```python
from build123d import *

# Parameters (mm, degrees)
F0_R     = 25.4
F0_R_2   = 12.7
F1_DEPTH = 3.175
F2_R     = 12.7
F3_DEPTH = 12.7


with BuildPart() as f1:
    # F0 (on Front) → F1 (new body)
    with BuildSketch(Plane.XZ):
        with Locations((-49.276002, 2.029355)):
            Circle(F0_R)
        with Locations((-49.276002, 2.029355)):
            Circle(F0_R_2, mode=Mode.SUBTRACT)
    extrude(amount=F1_DEPTH)

    # F2 (on face) → F3 (join)
    with BuildSketch(Plane.XZ.offset(3.175)):
        Polygon((-39.038599, -21.216195), (-24.026064, -0.727569), (-34.263467, 22.517981), (-59.513405, 25.274904), (-74.52594, 4.786278), (-64.288537, -18.459271), align=None)
        with Locations((-49.276002, 2.029355)):
            Circle(F2_R, mode=Mode.SUBTRACT)
    extrude(amount=F3_DEPTH)


solid = f1.part
```
Source: CAD feature listing. Evaluate the final solid. Frame: model axes, mm. A direction names the side the tool comes from. Coordinates: 2 decimals unless noted, no trailing zeros. Order: outer loops, then holes, each group sorted by start corner. A loop starts at its lowest first (then second) coordinate and runs counter-clockwise, first axis right, second up. Notation, with made-up numbers: (10.25, 75.5) - (68.25, 75.5) arc R16 ccw to (68.25, 94.5) - close; hole circle Ø2 at (40.25, 60). An arc over 180 degrees is marked (long way). One line per item, written item: value.
1) Ray query, line 1 (X direction, y = -11.5, z = -6); line 2 (Z direction, x = -42, y = -2.5); line 3 (Y direction, x = -28, z = -8.5) (3 decimals). Return the intervals inside material, ascending. Write a range as [from, to].
Computed values:
line 1: x = [-69.78, -59.12], [-39.44, -27.89]
line 2: z = [-22.31, -8.38], [12.44, 26.36]
line 3: y = [-3.175, 0]
2) Cut plane A-A on z = -2.5. Output: boundary loops of the cut face in (x, y) (3 decimals), plus the area to 3 significant figures.
Computed values:
outline: (-74.269, -3.175) - (-71.317, -3.175) - (-71.317, -15.875) - (-61.141, -15.875) - (-61.141, 0) - (-74.269, 0) - close; (-37.411, -15.875) - (-25.325, -15.875) - (-25.325, -3.175) - (-24.283, -3.175) - (-24.283, 0) - (-37.411, 0) - close
area: 366 mm^2
3) Cut plane B-B on x = -50. Output: boundary loops of the cut face in (y, z) (3 decimals).
Computed values:
outline: (-15.875, -20.019) - (-3.175, -20.019) - (-3.175, -23.36) - (0, -23.36) - (0, -10.65) - (-15.875, -10.65) - close; (-15.875, 14.709) - (0, 14.709) - (0, 27.419) - (-3.175, 27.419) - (-3.175, 24.236) - (-15.875, 24.236) - close
4) Cut plane D-D on x = -67. Output: boundary loops of the cut face in (y, z) (1 decimal).
Computed values:
outline: (-15.9, -12.3) - (-3.2, -12.3) - (-3.2, -16.2) - (0, -16.2) - (0, 20.2) - (-3.2, 20.2) - (-3.2, 15.1) - (-15.9, 15.1) - close
5) Reachability of faces 1 (the face through (-30, -3.175, -12)), 2 (the face through (-69.48, -9.44, -6.67)), 3 (the face through (-57.5, -3.175, 25.4)) from +Z, -Z, +X, -X, +Y, -Y: full face, straight path, thin tool, end or side. Return the list, or none.
Computed values:
face 1: -Z, +X, -Y
face 2: -Z, -X, -Y
face 3: +Z, -Y
6) Cut plane C-C on y = -9. Output: boundary loops of the cut face in (x, z).
Computed values:
outline: (-74.53, 4.79) - (-64.29, -18.46) - (-39.04, -21.22) - (-24.03, -0.73) - (-34.26, 22.52) - (-59.51, 25.27) - close; hole circle Ø25.4 at (-49.28, 2.03)
7) Contact query for flat-ended pins moving along their axis: pin 1 (1.5 mm diameter, centred on y = -6.5, z = -2, fed in from +X); pin 2 (1.5 mm diameter, centred on x = -65.5, y = -2.5, fed in from -Z); pin 3 (12 mm diameter, centred on x = -30, z = -14, fed in from -Y) (3 decimals); pin 4 (1.5 mm diameter, centred on x = -53, z = -21.5, fed in from -Y) (3 decimals). Output: stop coordinate, or through.
Computed values:
pin 1: stops at x = -24.41
pin 2: stops at z = -18.11
pin 3: stops at y = -15.875
pin 4: stops at y = -3.175
8) Mould query, pull axis X, two halves, no side actions, for faces 4 (the face through (-37.16, -7.83, 5.84)), 5 (the face through (-31.64, -9.44, -11.12)), 6 (the face through (-66.915, -9.436, 15.174)). Classes: released by +X, released by -X, zero draft, split by the parting line, or undercut.
Computed values:
face 4: undercut
face 5: released by +X
face 6: released by -X
